Verification items for this drawing (mm, ordinates from the low corner). Round coordinates to 2 decimals unless told otherwise and drop trailing zeros. Order: outer loops, then holes, each group sorted by start corner. A loop starts at its lowest first (then second) coordinate and runs counter-clockwise, first axis right, second up. Notation, with made-up numbers: (22.25, 3.5) - (33.25, 3.5) arc R21 cw to (33.25, 13.5) - close; hole circle Ø4 at (4.5, -24.5). An arc over 180 degrees is marked (long way). One line per question, with ' | ' between items. Start each with the question number.
Q1. Sectioned sample at C-C, the plane y = 11. Enter the section's corners in (x, z) (1 decimal).
Q2. Mould release check, pull along Z, two halves, no side actions. Record for the marked faces 1, 2, 3 and 4: +Z half, -Z half, draft (parallel to the pull), parting line (faces both ways), or undercut.
Q3. Material ranges on line 1 along Z through (x, y) = (22, 5.5) (1 decimal); line 2 along Z through (x, y) = (38, 13.5); line 3 along X through (y, z) = (37.5, 12), recorded low to high.
Q4. Gauge pin test, flat end, axial feed: P1, Ø10, axis at x = 31, z = 30.5, coming from the -Y side. Record the tip position at first contact, or that the pin passes through.
Q5. Sectioned sample at B-B, the plane z = 32. Enter the section's corners in (x, y), then the cut area to 3 significant figures.
Q6. Sectioned sample at A-A, the plane x = 39. Enter the section's corners in (y, z).
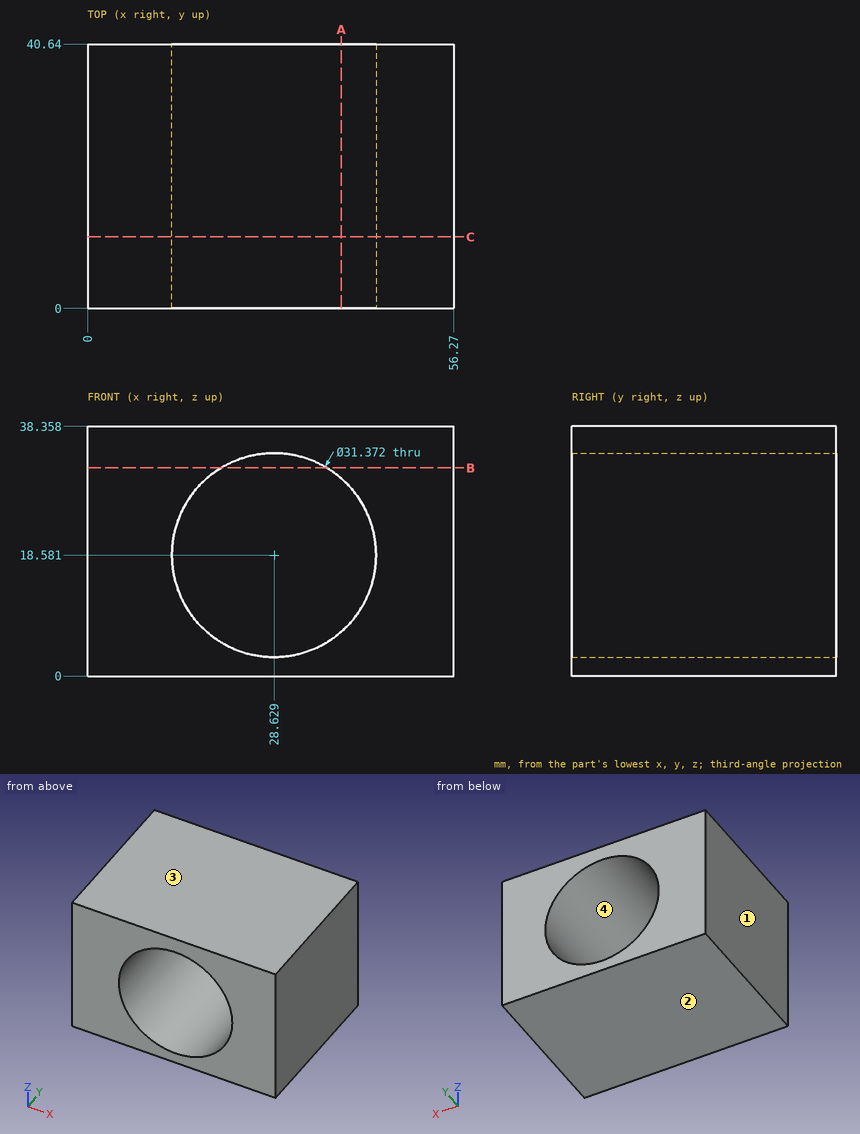
Determined:
1) outline: (0, 0) - (56.3, 0) - (56.3, 38.4) - (0, 38.4) - close; hole circle Ø31.4 at (28.6, 18.6)
2) face 1: draft | face 2: -Z half | face 3: +Z half | face 4: undercut
3) line 1: z = 0 to 4.4, 32.8 to 38.4 | line 2: z = 0 to 6, 31.16 to 38.36 | line 3: x = 0 to 14.39, 42.87 to 56.27
4) P1: stops at y = 0
5) outline: (0, 0) - (20.51, 0) - (20.51, 40.64) - (0, 40.64) - close; (36.75, 0) - (56.27, 0) - (56.27, 40.64) - (36.75, 40.64) - close | area: 1,630 mm2
6) outline: (0, 0) - (40.64, 0) - (40.64, 6.81) - (0, 6.81) - close; (0, 30.35) - (40.64, 30.35) - (40.64, 38.36) - (0, 38.36) - close
